```python
from build123d import *

# Parameters (mm, degrees)
SKETCH1_R           = 20
SKETCH1_R_2         = 2.1
BOSS_EXTRUDE1_DEPTH = 3
SKETCH2_R           = 5
BOSS_EXTRUDE2_DEPTH = 15
CUT_EXTRUDE1_START  = -12
CUT_EXTRUDE1_DEPTH  = 12


with BuildPart() as part:
    # Sketch1 → Boss-Extrude1 (new body)
    with BuildSketch(Plane(origin=(0, 0, 0), x_dir=(1, 0, 0), z_dir=(0, 1, 0))):
        with Locations(Location((0, 0, 0), (0, 0, 270))):
            Circle(SKETCH1_R)
        with Locations(Location((-14, 0, 0), (0, 0, 270))):
            Circle(SKETCH1_R_2, mode=Mode.SUBTRACT)
        with Locations(Location((0, 14, 0), (0, 0, 270))):
            Circle(SKETCH1_R_2, mode=Mode.SUBTRACT)
        with Locations(Location((14, 0, 0), (0, 0, 270))):
            Circle(SKETCH1_R_2, mode=Mode.SUBTRACT)
        with Locations(Location((0, -14, 0), (0, 0, 270))):
            Circle(SKETCH1_R_2, mode=Mode.SUBTRACT)
    extrude(amount=BOSS_EXTRUDE1_DEPTH)

    # Sketch2 → Boss-Extrude2 (add)
    with BuildSketch(Plane(origin=(0, 3, 0), x_dir=(1, 0, 0), z_dir=(0, 1, 0))):
        with Locations(Location((0, 0, 0), (0, 0, 270))):
            Circle(SKETCH2_R)
    extrude(amount=BOSS_EXTRUDE2_DEPTH)

    # Sketch3 → Cut-Extrude1 (cut)
    with BuildSketch(Plane(origin=(0, 18, 0), x_dir=(1, 0, 0), z_dir=(0, 1, 0)).offset(CUT_EXTRUDE1_START)):
        with BuildLine():
            Line((3.8, 3.249615362), (3.8, -3.249615362))
            ThreePointArc((3.8, -3.249615362), (5, 0), (3.8, 3.249615362))
        make_face()
    extrude(amount=CUT_EXTRUDE1_DEPTH, mode=Mode.SUBTRACT)


solid = part.part
```
The listing builds one solid part. Answer for the finished solid, in the listing's coordinates (mm). A direction names the side the tool comes from. Give positions to 0.01 mm unless a question says otherwise; leave off trailing zeros. Order: outer loops, then holes, each group sorted by start corner. A loop starts at its lowest first (then second) coordinate and runs counter-clockwise, first axis right, second up. Notation, with made-up numbers: (57.5, 12.25) - (113.5, 12.25) arc R19 cw to (113.5, 28.25) - close; hole circle Ø9 at (39, -25.5). An arc over 180 degrees is marked (long way). Answer in a Markdown table with one row per item. Add a question column.
Q1. Which of the six approach directions +Z, -Z, +X, -X, +Y, -Y give full straight-line access (tool end or side, diameter ignored) to faces 1 (the cylindrical face through (0.09, 1.48, 11.9)), 2 (the flat face through (-4, 3, 4)), 3 (the flat face through (3.8, 12, 0))?
Q2. The part is cut by section C-C (y = 2.5). Determine the outline of the cut face in (x, z).
Q3. The part is cut by section B-B (z = -13). Determine the outline of the cut face in (x, y), then the cut area to 3 significant figures.
Q4. The part is cut by section A-A (x = 0). Determine the outline of the cut face in (y, z), then the cut area to 3 significant figures.
Q5. The part is cut by section D-D (x = -14). Determine the outline of the cut face in (y, z).
Q6. Find the intervals of material crossed by line 1 along X through (y, z) = (0.8, 0); line 2 along Y through (x, z) = (9.5, -7); line 3 along X through (y, z) = (13.5, 1), in increasing order. Write a range as [from, to].
Q7. Given P1, Ø1, axis at x = -3, z = -14, coming from the +Y side; P2, Ø1.9, axis at y = 10, z = -1, coming from the +X side; P3, Ø3, axis at y = 2, z = -10, coming from the +X side, each flat-ended and moving along its own axis, determine where each tip first touches the part or whether it passes through.
Q8. For a pull along X with two mould halves and no side action, classify faces 4 (the flat face through (4, 6, 0)), 5 (the cylindrical face through (15.77, 1.48, 1.13)), 6 (the cylindrical face through (-19.524, 1.479, -4.336)) as released by +X, released by -X, zero draft, split by the parting line, or undercut.
Determined:
| question | item | result |
|---|---|---|
| 1 | face 1 | +Y, -Y |
| 1 | face 2 | +Y |
| 1 | face 3 | +Z, -Z, +X, +Y |
| 2 | outline | circle Ø40 at (0, 0); hole circle Ø4.2 at (-14, 0); hole circle Ø4.2 at (0, -14); hole circle Ø4.2 at (0, 14); hole circle Ø4.2 at (14, 0) |
| 3 | outline | (-15.2, 0) - (-1.85, 0) - (-1.85, 3) - (-15.2, 3) - close; (1.85, 0) - (15.2, 0) - (15.2, 3) - (1.85, 3) - close |
| 3 | area | 80.1 mm² |
| 4 | outline | (0, -20) - (3, -20) - (3, -16.1) - (0, -16.1) - close; (0, -11.9) - (3, -11.9) - (3, -5) - (18, -5) - (18, 5) - (3, 5) - (3, 11.9) - (0, 11.9) - close; (0, 16.1) - (3, 16.1) - (3, 20) - (0, 20) - close |
| 4 | area | 245 mm² |
| 5 | outline | (0, -14.28) - (3, -14.28) - (3, -2.1) - (0, -2.1) - close; (0, 2.1) - (3, 2.1) - (3, 14.28) - (0, 14.28) - close |
| 6 | line 1 | x = [-20, -16.1], [-11.9, 11.9], [16.1, 20] |
| 6 | line 2 | y = [0, 3] |
| 6 | line 3 | x = [-4.9, 3.8] |
| 7 | P1 | stops at y = 3 |
| 7 | P2 | stops at x = 3.8 |
| 7 | P3 | stops at x = 18.1 |
| 8 | face 4 | zero draft |
| 8 | face 5 | undercut |
| 8 | face 6 | split by the parting line |
